```python
from build123d import *

# Parameters (mm, degrees)
BOSS_EXTRUDE1_DEPTH = 2
BOSS_EXTRUDE2_DEPTH = 2
BOSS_EXTRUDE3_DEPTH = 106
SKETCH4_R           = 10
SKETCH4_R_2         = 6.55
BOSS_EXTRUDE4_DEPTH = 10
FILLET1_R           = 5
FILLET2_R           = 10


with BuildPart() as part:
    # Sketch1 → Boss-Extrude1 (new body)
    with BuildSketch(Plane.XY):
        Polygon((1, -21.742716482), (14.860117326, -21.742716482), (36, -42.882599156), (36, -121.742716482), (1, -121.742716482), align=None)
    extrude(amount=-BOSS_EXTRUDE1_DEPTH)



with BuildPart() as body_2:
    # Sketch2 → Boss-Extrude2 (new body)
    with BuildSketch(Plane(origin=(0, 0, -110), x_dir=(-1, 0, 0), z_dir=(0, 0, -1))):
        Polygon((-1, -121.742716482), (-1, -21.742716482), (-14.860117326, -21.742716482), (-36, -42.882599156), (-36, -121.742716482), align=None)
    extrude(amount=-BOSS_EXTRUDE2_DEPTH)


with BuildPart() as part_1:
    add(part.part)

    add(body_2.part)  # Boss-Extrude3 merges body 2
    # Sketch3 → Boss-Extrude3 (add)
    with BuildSketch(Plane(origin=(0, 0, -2), x_dir=(-1, 0, 0), z_dir=(0, 0, -1))):
        Polygon((-1, -23.742716482), (-14.031690201, -23.742716482), (-34, -43.71102628), (-34, -119.742716482), (-1, -119.742716482), (-1, -121.742716482), (-36, -121.742716482), (-36, -42.882599156), (-14.860117326, -21.742716482), (-1, -21.742716482), align=None)
    extrude(amount=BOSS_EXTRUDE3_DEPTH)

    # Sketch4 → Boss-Extrude4 (add)
    with BuildSketch(Plane(origin=(36, 0, 0), x_dir=(0, 0, -1), z_dir=(1, 0, 0))):
        with Locations(Location((20, -82.312657819, 0), (0, 0, 90))):
            Circle(SKETCH4_R)
        with Locations(Location((20, -82.312657819, 0), (0, 0, 90))):
            Circle(SKETCH4_R_2, mode=Mode.SUBTRACT)
    extrude(amount=BOSS_EXTRUDE4_DEPTH)

    # Fillet1
    fillet1_edges = [part_1.edges().sort_by_distance(p)[0] for p in [
        (17.5, -119.742716482, -2),
        (17.5, -119.742716482, -108),
        (18.5, -121.742716482, -110),
        (18.5, -121.742716482, 0),
    ]]
    fillet(fillet1_edges, radius=FILLET1_R)

    # Fillet2
    fillet2_edges = [part_1.edges().sort_by_distance(p)[0] for p in [
        (34, -43.71102628, -55),
        (14.031690201, -23.742716482, -55),
        (14.860117326, -21.742716482, -55),
        (36, -42.882599156, -55),
    ]]
    fillet(fillet2_edges, radius=FILLET2_R)


solid = part_1.part
```
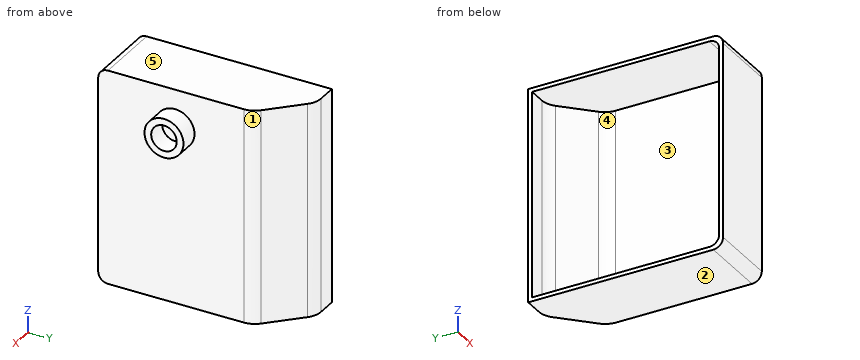
Work out the finished part from the listing and answer in its coordinate system (mm). Face numbers are marked on the shaded views. A direction names the side the tool comes from. Give positions to 0.01 mm unless a question says otherwise; leave off trailing zeros. Write each loop counter-clockwise with the first axis right and the second up, starting at its lowest first coordinate (ties: lowest second). Pieces come first, ordered by that corner, then holes. Notation, with made-up numbers: (76, 50.25) -> (100, 50.25) arc R21 cw to (100, 73.25) -> close; hole circle Ø6 at (47, 35.25). An arc over 180 degrees is marked (long way). Write each question's results on one line, items separated by ' | '.
1. Find section B-B on z = -20. Determine the outline of the cut face in (x, y), and give its area (3 significant figures).
Data:
outline: (1, -121.74) -> (36, -121.74) -> (36, -92.31) -> (46, -92.31) -> (46, -88.86) -> (36, -88.86) -> (36, -75.76) -> (46, -75.76) -> (46, -72.31) -> (36, -72.31) -> (36, -47.02) arc R10 ccw to (33.07, -39.95) -> (17.79, -24.67) arc R10 ccw to (10.72, -21.74) -> (1, -21.74) -> (1, -23.74) -> (9.89, -23.74) arc R10 cw to (16.96, -26.67) -> (31.07, -40.78) arc R10 cw to (34, -47.85) -> (34, -119.74) -> (1, -119.74) -> close | area: 377 mm^2
2. Each of these flat-tipped pins is pushed along its axis until it touches: pin 1 Ø21 at (y, z) = (-82.31, -20) entering from -X; pin 2 Ø6.5 at (y, z) = (-84, -22.5) entering from +X; pin 3 Ø1 at (x, z) = (37, -60) entering from -Y. Where does it stop, or does it pass through?
Data:
pin 1: x = 34 | pin 2: x = 36 | pin 3: through
3. Straight lines are drawn through the part: L1, parallel to Z at x = 23.5, y = -38; L2, parallel to Y at x = 8.5, z = -47; L3, parallel to X at y = -79, z = -59. For each, find the intervals that lie inside material, in ascending order.
Data:
L1: -110 to -108, -2 to 0 | L2: -121.74 to -119.74, -23.74 to -21.74 | L3: 34 to 36
4. A tool of negligible diameter and unlimited length cuts with its end or side. For the marked faces 4 and 5, from which of +Z, -Z, +X, -X, +Y, -Y can it reach the whole face along a straight path? Write none if from no direction.
Data:
face 4: -X | face 5: +Z, +X, -X, +Y, -Y
5. Find section A-A on x = 8.5. Determine the outline of the cut face in (y, z).
Data:
outline: (-121.74, -105) arc R5 ccw to (-116.74, -110) -> (-21.74, -110) -> (-21.74, 0) -> (-116.74, 0) arc R5 ccw to (-121.74, -5) -> close; hole (-119.74, -103) arc R5 ccw to (-114.74, -108) -> (-23.74, -108) -> (-23.74, -2) -> (-114.74, -2) arc R5 ccw to (-119.74, -7) -> close
6. Determine the mould class of the marked faces 1, 2 and 3 for opening direction Y: +Y half, -Y half, draft (parallel to the pull), parting line (faces both ways), or undercut.
Data:
face 1: +Y half | face 2: draft | face 3: undercut
7. Find section D-D on z = -44. Determine the outline of the cut face in (x, y).
Data:
outline: (1, -121.74) -> (36, -121.74) -> (36, -47.02) arc R10 ccw to (33.07, -39.95) -> (17.79, -24.67) arc R10 ccw to (10.72, -21.74) -> (1, -21.74) -> (1, -23.74) -> (9.89, -23.74) arc R10 cw to (16.96, -26.67) -> (31.07, -40.78) arc R10 cw to (34, -47.85) -> (34, -119.74) -> (1, -119.74) -> close
8. Find section C-C on y = -95. Determine the outline of the cut face in (x, z).
Data:
outline: (1, -110) -> (36, -110) -> (36, 0) -> (1, 0) -> (1, -2) -> (34, -2) -> (34, -108) -> (1, -108) -> close
